The drawing under review shows one solid part. Ordinate dimensions are in mm from its lowest x, y, z. A direction names the side the tool comes from. Coordinates: 2 decimals unless noted, no trailing zeros. Loops run counter-clockwise (first coordinate to the right, second up) from the corner with the lowest first, then second, coordinate; pieces in that order, holes last. Notation, with made-up numbers: M 82.5,-14 L 126.5,-14 A24 cw 126.5,14 Z; hole C -3,-35.75 d10. An arc over 180 degrees is marked long. Answer as a JSON object with one key per item and string values. Group by question number.
1. Consider section A-A (z = 10.25). State the section outline as (x, y) points.
2. Consider section B-B (y = 26.5). State the section outline as (x, z) points, then the cut area to 3 significant figures.
3. Consider section C-C (x = 25). State the section outline as (y, z) points.
4. To check wall thickness, follow probe 1 along Z at (x, y) = (30, 20.5); probe 2 along X at (y, z) = (17, 6.5); probe 3 along Z at (x, y) = (31.5, 27). State the ranges of each line that lie inside material, in increasing order.
5. Machinability: for the marked faces 1, 2 and 3, which of the approach directions +Z, -Z, +X, -X, +Y, -Y give a long, thin tool a straight path to every point of the face, cutting with its end or side? Answer none if there is none.
6. Insertion check: pin 1 (5 mm diameter, centred on y = 28, z = 20.5, fed in from -X); pin 2 (3 mm diameter, centred on y = 6, z = 19, fed in from +X); pin 3 (5 mm diameter, centred on x = 3, z = 11.5, fed in from +Y). Each pin has a flat end and moves straight along its axis. Give the tip position at first contact, or say it passes through.
7. Consider section D-D (x = 58). State the section outline as (y, z) points.
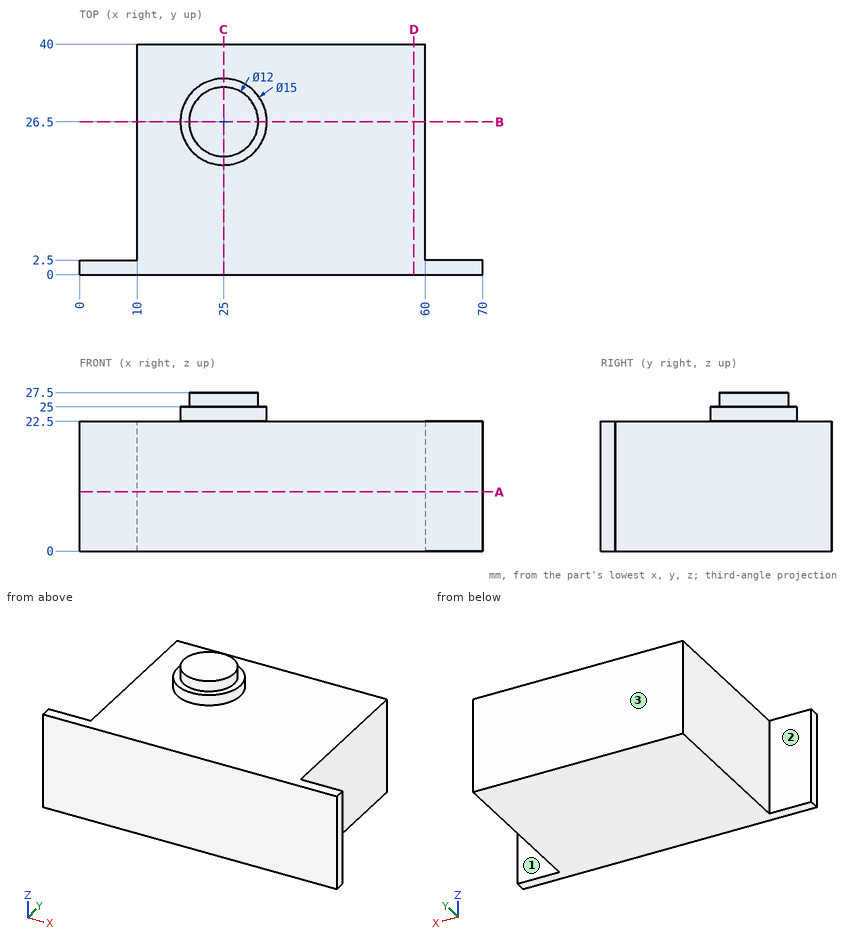
Findings below:
{
 "1": {"outline": "M 0,0 L 70,0 L 70,2.5 L 60,2.5 L 60,40 L 10,40 L 10,2.5 L 0,2.5 Z"},
 "2": {"outline": "M 10,0 L 60,0 L 60,22.5 L 32.5,22.5 L 32.5,25 L 31,25 L 31,27.5 L 19,27.5 L 19,25 L 17.5,25 L 17.5,22.5 L 10,22.5 Z", "area": "1,190 mm^2"},
 "3": {"outline": "M 0,0 L 40,0 L 40,22.5 L 34,22.5 L 34,25 L 32.5,25 L 32.5,27.5 L 20.5,27.5 L 20.5,25 L 19,25 L 19,22.5 L 0,22.5 Z"},
 "4": {"probe 1": "z = 0 to 22.5", "probe 2": "x = 10 to 60", "probe 3": "z = 0 to 25"},
 "5": {"face 1": "+Z, -Z, +X, +Y", "face 2": "+Z, -Z, -X, +Y", "face 3": "+Z, -Z, +X, -X, +Y"},
 "6": {"pin 1": "stops at x = 10", "pin 2": "stops at x = 60", "pin 3": "stops at y = 2.5"},
 "7": {"outline": "M 0,0 L 40,0 L 40,22.5 L 0,22.5 Z"}
}
